The model under review builds one solid part; all positions refer to its coordinate system, in mm. Give positions to 0.01 mm unless a question says otherwise; leave off trailing zeros. Write each loop counter-clockwise with the first axis right and the second up, starting at its lowest first coordinate (ties: lowest second). Pieces come first, ordered by that corner, then holes. Notation, with made-up numbers: (-37, 7) - (-15, 7) arc R12 ccw to (-15, 29) - close; hole circle Ø10 at (-1, 50). An arc over 180 degrees is marked (long way). Write item = value, one per line.
Autodesk Inventor part; units mm, degrees
ref_plane "YZ Plane" through (0, 0, 0) normal (1, 0, 0) x (0, 1, 0)
ref_plane "XZ Plane" through (0, 0, 0) normal (0, 1, 0) x (-1, 0, 0)
ref_plane "XY Plane" through (0, 0, 0) normal (0, 0, 1) x (1, 0, 0)
sketch "Sketch1" plane through (0, 0, 0) normal (0, 0, 1) x (1, 0, 0)
  line L0 (-7.5, 5) -> (7.5, 5)
  line L1 (7.5, 5) -> (7.5, -5)
  line L2 (7.5, -5) -> (-7.5, -5)
  line L3 (-7.5, -5) -> (-7.5, 5)
  line L4 (-7.5, 5) -> (7.5, -5) construction
  line L5 (7.5, 5) -> (-7.5, -5) construction
  line L6 (-7.5, 3.0607) -> (-6.4393, 2)
  line L7 (-7.5, 3.0607) -> (-6, 3.0607) construction
  line L8 (-6.4393, 2) -> (-7.5, 0.9393)
  line L9 (0, 5) -> (0, -5) construction
  line L10 (7.5, 3.0607) -> (6.4393, 2)
  line L11 (6.4393, 2) -> (7.5, 0.9393)
  point P0 (0, 0)
  point P1 (7.5, 0.9393)
  point P2 (7.5, 3.0607)
  dimension "d0" = 15
  dimension "d1" = 10
  dimension "d2" = 45
  dimension "d3" = 3
  dimension "d4" = 1.5
extrude "Extrusion1" add sketch "Sketch1" along normal mid plane 360 contours L0 L1 L10 L11 L2 L3 L8 L6
sketch "Sketch2" plane through (-7.5, 5, 180) normal (0, 1, 0) x (1, 0, 0)
  point P0 (7.5, 180)
  point P1 (7.5, 180)
hole "Hole1" at (0, 5, 0) direction (0, -1, 0) diameter 3.5 end through all counterbore diameter 6 counterbore depth 4.5
pattern_linear "Rectangular Pattern1" count 9 spacing 40 along (0, 0, 1) of "Hole1" first direction both ways yes
sketch "Sketch3" plane through (-7.5, 5, 180) normal (0, 1, 0) x (1, 0, 0)
  point P0 (7.5, 180)
  point P1 (7.5, 180)
hole "Hole2" at (0, 5, 0) direction (0, -1, 0) diameter 6 end through all
sketch "Sketch4" plane through (0, 0, 180) normal (0, 0, 1) x (1, 0, 0)
  line L0 (-7.5, 5) -> (-7.5, 3.0607)
  line L1 (-7.5, 3.0607) -> (-6.4393, 2)
  line L2 (-6.4393, 2) -> (-7.5, 0.9393)
  line L3 (-7.5, 0.9393) -> (-7.5, -5)
  line L4 (-7.5, -5) -> (7.5, -5)
  line L5 (7.5, -5) -> (7.5, 0.9393)
  line L6 (7.5, 0.9393) -> (6.4393, 2)
  line L7 (6.4393, 2) -> (7.5, 3.0607)
  line L8 (7.5, 3.0607) -> (7.5, 5)
  line L9 (7.5, 5) -> (-7.5, 5)
  point P0 (0, 0)
extrude "Extrusion2" cut sketch "Sketch4" against normal blind 4.25
sketch "Sketch5" plane through (0, 0, -180) normal (0, 0, -1) x (-1, 0, 0)
  line L0 (7.5, 3.0607) -> (7.5, 5)
  line L1 (7.5, 5) -> (-7.5, 5)
  line L2 (-7.5, 5) -> (-7.5, 3.0607)
  line L3 (-7.5, 3.0607) -> (-6.4393, 2)
  line L4 (-6.4393, 2) -> (-7.5, 0.9393)
  line L5 (-7.5, 0.9393) -> (-7.5, -5)
  line L6 (-7.5, -5) -> (7.5, -5)
  line L7 (7.5, -5) -> (7.5, 0.9393)
  line L8 (7.5, 0.9393) -> (6.4393, 2)
  line L9 (6.4393, 2) -> (7.5, 3.0607)
  point P0 (0, 0)
extrude "Extrusion3" cut sketch "Sketch5" against normal blind 1.25
properties part number "MGN15 Rail" material "Stainless Steel, 440C"
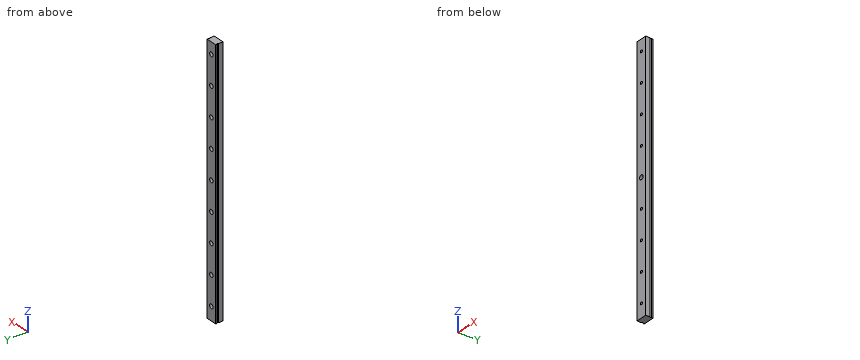
1. Take a section at A-A on z = -109. Give the boundary of the cut face in (x, y), and give its area (3 significant figures).
Findings below:
outline = (-7.5, -5) - (7.5, -5) - (7.5, 0.94) - (6.44, 2) - (7.5, 3.06) - (7.5, 5) - (-7.5, 5) - (-7.5, 3.06) - (-6.44, 2) - (-7.5, 0.94) - close
area = 148 mm²
2. Take a section at C-C on z = 0. Give the boundary of the cut face in (x, y), and give its area (4 significant figures).
Findings below:
outline = (-7.5, -5) - (-3, -5) - (-3, 5) - (-7.5, 5) - (-7.5, 3.06) - (-6.44, 2) - (-7.5, 0.94) - close; (3, -5) - (7.5, -5) - (7.5, 0.94) - (6.44, 2) - (7.5, 3.06) - (7.5, 5) - (3, 5) - close
area = 87.75 mm²
3. For line 1 (X direction, y = 3, z = -40.5); line 2 (X direction, y = -1.1, z = -160); line 3 (Y direction, x = -0.25, z = -77.5), list the stretches that pass through material, from the lowest coordinate up. Write a range as from..to.
Findings below:
line_1 = -7.44..-2.96, 2.96..7.44
line_2 = -7.5..-1.75, 1.75..7.5
line_3 = -5..0.5
4. Insertion check: P1, Ø1.8, axis at x = 0.5, z = 40.5, coming from the +Y side; P2, Ø1.8, axis at x = -0.5, z = 121, coming from the +Y side. Each pin has a flat end and moves straight along its axis. Give the tip position at first contact, or say it passes through.
Findings below:
P1 = through
P2 = 0.5
5. Take a section at B-B on y = -2.5. Count the separate pieces of the cut face and the enclosed holes in it, and give its area (3 significant figures).
Findings below:
separate_pieces = 1
enclosed_holes = 9
area = 5,210 mm²
